Geometry: final body of the model. Coordinates: model frame, mm. A direction names the side the tool comes from. Round coordinates to 2 decimals unless told otherwise and drop trailing zeros. Loops run counter-clockwise (first coordinate to the right, second up) from the corner with the lowest first, then second, coordinate; pieces in that order, holes last. Notation, with made-up numbers: M 54,17.5 L 84,17.5 A17 ccw 84,33.5 Z; hole C -32.75,-4 d1. An arc over 180 degrees is marked long. Write each question's results on one line, items separated by ' | '.
Autodesk Inventor part; units mm, degrees
ref_plane "YZ Plane" through (0, 0, 0) normal (1, 0, 0) x (0, 1, 0)
ref_plane "XZ Plane" through (0, 0, 0) normal (0, 1, 0) x (-1, 0, 0)
ref_plane "XY Plane" through (0, 0, 0) normal (0, 0, 1) x (1, 0, 0)
sketch "スケッチ1" plane through (0, 0, 0) normal (0, 0, 1) x (1, 0, 0)
  line L0 (0, 0) -> (40, 0)
  line L1 (40, 0) -> (40, 50)
  line L2 (40, 50) -> (0, 50)
  line L3 (0, 50) -> (0, 0)
  dimension "d0" = 40
  dimension "d1" = 50
extrude "押し出し1" add sketch "スケッチ1" along normal blind 3
sketch "スケッチ2" plane through (0, 0, 3) normal (0, 0, 1) x (1, 0, 0)
  line L0 (40, 50) -> (0, 50)
  line L1 (40, 0) -> (40, 50)
  line L2 (0, 50) -> (40, 50)
  line L3 (40, 50) -> (40, 47)
  line L4 (40, 47) -> (0, 47)
  line L5 (0, 47) -> (0, 50)
  line L6 (0, 50) -> (0, 0)
  line L7 (0, 0) -> (40, 0)
  line L8 (40, 0) -> (40, 3)
  line L9 (40, 3) -> (0, 3)
  line L10 (0, 3) -> (0, 0)
  point P0 (0, 3)
  dimension "d5" = 3
  dimension "d6" = 3
extrude "押し出し2" add sketch "スケッチ2" along normal blind 27 contours L1 L4 L5 L0 | L1 L7 L6 L9
sketch "スケッチ3" plane through (0, 50, 0) normal (0, 1, 0) x (1, 0, 0)
  line L0 (0, 0) -> (0, -30)
  line L1 (40, 0) -> (0, 0)
  point P0 (20, -18)
  dimension "d9" = 20
  dimension "d10" = 18
hole "穴1" at (20, 50, 18) direction (0, -1, 0) diameter 10 depth 3
sketch "スケッチ5" plane through (0, 0, 0) normal (0, -1, 0) x (1, 0, 0)
  line L0 (40, 0) -> (40, 30)
  line L1 (40, 15) -> (0, 15)
  line L2 (0, 3) -> (0, 30)
  line L3 (0, 0) -> (40, 0)
  line L4 (20, 0) -> (20, 30)
  line L5 (0, 30) -> (40, 30)
  point P0 (25, 1.5)
  point P1 (15, 1.5)
  point P2 (25, 28.5)
  point P3 (15, 28.5)
  dimension "d18" = 10
  dimension "d19" = 27
hole "穴2" at (25, 0, 1.5) at (15, 0, 1.5) at (25, 0, 28.5) at (15, 0, 28.5) direction (0, 1, 0) diameter 1.567 depth 4 tip angle 118
sketch "スケッチ6" plane through (0, 50, 0) normal (0, 1, 0) x (1, 0, 0)
  line L0 (40, 0) -> (0, 0)
  line L1 (20, 0) -> (20, -30)
  line L2 (40, -30) -> (0, -30)
  line L3 (0, 0) -> (0, -30)
  line L4 (0, -15) -> (40, -15)
  line L5 (40, 0) -> (40, -30)
  point P0 (5, -5)
  point P1 (35, -5)
  point P2 (5, -25)
  point P3 (35, -25)
  dimension "d27" = 20
  dimension "d28" = 30
hole "穴3" at (5, 50, 5) at (35, 50, 5) at (5, 50, 25) at (35, 50, 25) direction (0, -1, 0) diameter 2.459 depth 3
fillet "フィレット1" radius 2 4 edges at (0, 48.5, 30) (0, 1.5, 30) (40, 48.5, 30) (40, 1.5, 30)
properties part number "arm" material "アルミニウム 6061"
1. Section C-C (z = 25). Output: boundary loops of the cut face in (x, y).
Answer key:
outline: M 0,0 L 40,0 L 40,3 L 0,3 Z; M 0,47 L 3.77,47 L 3.77,50 L 0,50 Z; M 6.23,47 L 33.77,47 L 33.77,50 L 6.23,50 Z; M 36.23,47 L 40,47 L 40,50 L 36.23,50 Z
2. Ray query, probe 1 along X at (y, z) = (48.6, 5); probe 2 along Z at (x, y) = (35, 48); probe 3 along Z at (x, y) = (15, 2.3). Return the intervals inside material, ascending.
Answer key:
probe 1: x = 0 to 3.77, 6.23 to 33.77, 36.23 to 40 | probe 2: z = 0 to 3.77, 6.23 to 23.77, 26.23 to 30 | probe 3: z = 0 to 0.72, 2.28 to 27.72, 29.28 to 30
3. Pin query (flat end, axial travel): P1, Ø3, axis at y = 33.5, z = 5, coming from the -X side; P2, Ø20, axis at x = 12.5, y = 25, coming from the +Z side; P3, Ø0.9, axis at x = 25, z = 28.5, coming from the -Y side; P4, Ø2, axis at x = 5, z = 5, coming from the +Y side. Return the tip coordinate at first contact, or that it passes through.
Answer key:
P1: passes through | P2: stops at z = 3 | P3: stops at y = 47 | P4: stops at y = 3
4. Draft query along Z for faces 4 (the face through (20, 3, 16)), 5 (the face through (20, 2, 30)), 6 (the face through (33.78, 48.48, 4.84)). Return one class per face: pulls with the +Z half, pulls with the -Z half, needs draft (parallel to the pull), parting line crosses it, or undercut.
Answer key:
face 4: needs draft | face 5: pulls with the +Z half | face 6: undercut
5. Section A-A (x = 35). Output: boundary loops of the cut face in (y, z), then the cut area to 3 significant figures.
Answer key:
outline: M 0,0 L 50,0 L 50,3.77 L 47,3.77 L 47,3 L 3,3 L 3,30 L 0,30 Z; M 47,6.23 L 50,6.23 L 50,23.77 L 47,23.77 Z; M 47,26.23 L 50,26.23 L 50,30 L 47,30 Z | area: 297 mm²
6. Access query for faces 1 (the face through (0.6, 1.48, 29.43)), 2 (the face through (14.765, 2.028, 0.753)), 3 (the face through (24.88, 48.48, 16.92)). Directions: +Z, -Z, +X, -X, +Y, -Y. A direction counts if a zero-diameter tool reaches every point of the face in a straight line with its end or side. Return the directions, or none.
Answer key:
face 1: +Z, -X, +Y, -Y | face 2: -Y | face 3: +Y
7. Section D-D (z = 18). Output: boundary loops of the cut face in (x, y), then the cut area to 3 significant figures.
Answer key:
outline: M 0,0 L 40,0 L 40,3 L 0,3 Z; M 0,47 L 15,47 L 15,50 L 0,50 Z; M 25,47 L 40,47 L 40,50 L 25,50 Z | area: 210 mm²
8. Section B-B (z = 12.25). Output: boundary loops of the cut face in (x, y).
Answer key:
outline: M 0,0 L 40,0 L 40,3 L 0,3 Z; M 0,47 L 40,47 L 40,50 L 0,50 Z
